The listing builds one solid part. Answer for the finished solid, in the listing's coordinates (mm). A direction names the side the tool comes from. Coordinates: 2 decimals unless noted, no trailing zeros. Order: outer loops, then holes, each group sorted by start corner. A loop starts at its lowest first (then second) coordinate and runs counter-clockwise, first axis right, second up. Notation, with made-up numbers: (81, 68) -> (130, 68) arc R28 ccw to (130, 92) -> close; hole circle Ø4 at (12, 89). An arc over 180 degrees is marked (long way). Answer in a Markdown table with one row per item.
```python
from build123d import *

# Parameters (mm, degrees)
F1_DEPTH = 12.7


with BuildPart() as f1:
    # F0 (on Top) → F1 (new body)
    with BuildSketch(Plane.XY):
        with BuildLine():
            ThreePointArc((0.353553, -0.353553), (-0.5, 0), (0.353553, 0.353553))
            Line((0.353553, 0.353553), (2.54, 2.54))
            Line((2.54, 2.54), (11.696242, 2.54))
            Line((11.696242, 2.54), (20.066, 2.54))
            Line((20.066, 2.54), (22.252447, 0.353553))
            ThreePointArc((22.252447, 0.353553), (23.106, 0), (22.252447, -0.353553))
            Line((22.252447, -0.353553), (20.066, -2.54))
            ThreePointArc((20.066, -2.54), (19.849227, -3.62979), (20.773107, -4.247107))
            Line((20.773107, -4.247107), (23.336, -4.247107))
            ThreePointArc((23.336, -4.247107), (24.234026, -3.875132), (24.606, -2.977107))
            Line((24.606, -2.977107), (24.606, 0))
            ThreePointArc((24.606, 0), (24.453759, 0.765367), (24.020214, 1.414214))
            Line((24.020214, 1.414214), (20.894427, 4.54))
            Line((20.894427, 4.54), (11.696242, 4.54))
            Line((11.696242, 4.54), (1.711573, 4.54))
            Line((1.711573, 4.54), (-1.414214, 1.414214))
            ThreePointArc((-1.414214, 1.414214), (-1.847759, 0.765367), (-2, 0))
            Line((-2, 0), (-2, -2.977107))
            ThreePointArc((-2, -2.977107), (-1.628026, -3.875132), (-0.73, -4.247107))
            Line((-0.73, -4.247107), (1.832893, -4.247107))
            ThreePointArc((1.832893, -4.247107), (2.756773, -3.62979), (2.54, -2.54))
            Line((2.54, -2.54), (0.353553, -0.353553))
        make_face()
    extrude(amount=F1_DEPTH)


solid = f1.part
```
(1) A cutting plane is placed at B-B, the plane x = 0. Determine the outline of the cut face in (y, z), then the cut area to 3 significant figures.
Check values:
| item | result |
|---|---|
| outline | (-4.25, 0) -> (-0.5, 0) -> (-0.5, 12.7) -> (-4.25, 12.7) -> close; (0.5, 0) -> (2.83, 0) -> (2.83, 12.7) -> (0.5, 12.7) -> close |
| area | 77.2 mm² |
(2) A cutting plane is placed at A-A, the plane y = 2. Determine the outline of the cut face in (x, z).
Check values:
| item | result |
|---|---|
| outline | (-0.83, 0) -> (2, 0) -> (2, 12.7) -> (-0.83, 12.7) -> close; (20.61, 0) -> (23.43, 0) -> (23.43, 12.7) -> (20.61, 12.7) -> close |
(3) A cutting plane is placed at C-C, the plane z = 2. Determine the outline of the cut face in (x, y), then the cut area to 3 significant figures.
Check values:
| item | result |
|---|---|
| outline | (-2, -2.98) arc R1.27 ccw to (-0.73, -4.25) -> (1.83, -4.25) arc R1 ccw to (2.54, -2.54) -> (0.35, -0.35) arc R0.5 cw (long way) to (0.35, 0.35) -> (2.54, 2.54) -> (20.07, 2.54) -> (22.25, 0.35) arc R0.5 cw (long way) to (22.25, -0.35) -> (20.07, -2.54) arc R1 ccw to (20.77, -4.25) -> (23.34, -4.25) arc R1.27 ccw to (24.61, -2.98) -> (24.61, 0) arc R2 ccw to (24.02, 1.41) -> (20.89, 4.54) -> (1.71, 4.54) -> (-1.41, 1.41) arc R2 ccw to (-2, 0) -> close |
| area | 86.6 mm² |
(4) Which of the six approach directions +Z, -Z, +X, -X, +Y, -Y give full straight-line access (tool end or side, diameter ignored) to faces 1 (the flat face through (21.144, 1.462, 6.261)), 2 (the cylindrical face through (-1.84, 0.78, 6.26))?
Check values:
| item | result |
|---|---|
| face 1 | +Z, -Z |
| face 2 | +Z, -Z, -X, +Y |
(5) For a pull along X with two mould halves and no side action, classify faces 3 (the cylindrical face through (-0.5, 0, 6.3)), 4 (the flat face through (11, 3, 0)), 5 (the flat face through (24.606, -2, 6)) as released by +X, released by -X, zero draft, split by the parting line, or undercut.
Check values:
| item | result |
|---|---|
| face 3 | undercut |
| face 4 | zero draft |
| face 5 | released by +X |
(6) A cutting plane is placed at D-D, the plane x = 17. Determine the outline of the cut face in (y, z), then the cut area to 3 significant figures.
Check values:
| item | result |
|---|---|
| outline | (2.54, 0) -> (4.54, 0) -> (4.54, 12.7) -> (2.54, 12.7) -> close |
| area | 25.4 mm² |
(7) Find the intervals of material crossed by line 1 along X through (y, z) = (0, 7); line 2 along Y through (x, z) = (0, 5.5); line 3 along Y through (x, z) = (15, 8.5), in increasing order. Write a range as from..to.
Check values:
| item | result |
|---|---|
| line 1 | -2..-0.5, 23.11..24.61 |
| line 2 | -4.25..-0.5, 0.5..2.83 |
| line 3 | 2.54..4.54 |
